```python
from build123d import *

# Parameters (mm, degrees)
SKETCH_1_W              = 150
SKETCH_1_H              = 200
EXTRUDE_1_DEPTH         = 2
CUT_EXTRUDE_1_REACH     = 127.016
SKETCH_2_R              = 2
CUT_EXTRUDE_2_REACH     = 127.016
SKETCH_3_R              = 1.6
CUT_EXTRUDE_3_REACH     = 127.016
SKETCH_5_R              = 1.6
CUT_EXTRUDE_START       = -2
CUT_EXTRUDE_4_OUTLINE_W = 150
CUT_EXTRUDE_4_OUTLINE_H = 200
CUT_EXTRUDE_4_DEPTH     = 2


# Read off the part's stored shape, not the designer's step: 切除-拉伸4
with BuildPart() as part:
    # 草图1 → 凸台-拉伸1 (new body)
    with BuildSketch(Plane(origin=(0, 0, 0), x_dir=(1, 0, 0), z_dir=(0, 1, 0))):
        Rectangle(SKETCH_1_W, SKETCH_1_H)
    extrude(amount=EXTRUDE_1_DEPTH)

    # 草图2 → 切除-拉伸1 (cut, up to next)
    with BuildSketch(Plane(origin=(0, 2, 0), x_dir=(1, 0, 0), z_dir=(0, 1, 0)), mode=Mode.PRIVATE) as cut_extrude_1_sk1:
        with Locations(Location((0, 80, 0), (0, 0, 270))):
            Circle(SKETCH_2_R)
    cut_extrude_1_tool1 = extrude(cut_extrude_1_sk1.sketch, amount=-CUT_EXTRUDE_1_REACH, mode=Mode.PRIVATE) & part.part
    add(cut_extrude_1_tool1.solids().sort_by_distance((0, 2, -80))[0], mode=Mode.SUBTRACT)

    # 草图3 → 切除-拉伸2 (cut, up to next)
    with BuildSketch(Plane(origin=(0, 2, 0), x_dir=(1, 0, 0), z_dir=(0, 1, 0)), mode=Mode.PRIVATE) as cut_extrude_2_sk1:
        with Locations(Location((-17.5, 35, 0), (0, 0, 270))):
            Circle(SKETCH_3_R)
    cut_extrude_2_tool1 = extrude(cut_extrude_2_sk1.sketch, amount=-CUT_EXTRUDE_2_REACH, mode=Mode.PRIVATE) & part.part
    # 草图3 → 切除-拉伸2 (cut, up to next)
    with BuildSketch(Plane(origin=(0, 2, 0), x_dir=(1, 0, 0), z_dir=(0, 1, 0)), mode=Mode.PRIVATE) as cut_extrude_2_sk2:
        with Locations(Location((-17.5, 25, 0), (0, 0, 90))):
            Circle(SKETCH_3_R)
    cut_extrude_2_tool2 = extrude(cut_extrude_2_sk2.sketch, amount=-CUT_EXTRUDE_2_REACH, mode=Mode.PRIVATE) & part.part
    # 草图3 → 切除-拉伸2 (cut, up to next)
    with BuildSketch(Plane(origin=(0, 2, 0), x_dir=(1, 0, 0), z_dir=(0, 1, 0)), mode=Mode.PRIVATE) as cut_extrude_2_sk3:
        with Locations(Location((17.5, 25, 0), (0, 0, 270))):
            Circle(SKETCH_3_R)
    cut_extrude_2_tool3 = extrude(cut_extrude_2_sk3.sketch, amount=-CUT_EXTRUDE_2_REACH, mode=Mode.PRIVATE) & part.part
    # 草图3 → 切除-拉伸2 (cut, up to next)
    with BuildSketch(Plane(origin=(0, 2, 0), x_dir=(1, 0, 0), z_dir=(0, 1, 0)), mode=Mode.PRIVATE) as cut_extrude_2_sk4:
        with Locations(Location((17.5, 35, 0), (0, 0, 90))):
            Circle(SKETCH_3_R)
    cut_extrude_2_tool4 = extrude(cut_extrude_2_sk4.sketch, amount=-CUT_EXTRUDE_2_REACH, mode=Mode.PRIVATE) & part.part
    add(cut_extrude_2_tool1.solids().sort_by_distance((-17.5, 2, -35))[0], mode=Mode.SUBTRACT)
    add(cut_extrude_2_tool2.solids().sort_by_distance((-17.5, 2, -25))[0], mode=Mode.SUBTRACT)
    add(cut_extrude_2_tool3.solids().sort_by_distance((17.5, 2, -25))[0], mode=Mode.SUBTRACT)
    add(cut_extrude_2_tool4.solids().sort_by_distance((17.5, 2, -35))[0], mode=Mode.SUBTRACT)

    # 草图5 → 切除-拉伸3 (cut, up to next)
    with BuildSketch(Plane(origin=(0, 2, 0), x_dir=(1, 0, 0), z_dir=(0, 1, 0)), mode=Mode.PRIVATE) as cut_extrude_3_sk1:
        with Locations(Location((32.32051615, -5, 0), (0, 0, 270))):
            Circle(SKETCH_5_R)
    cut_extrude_3_tool1 = extrude(cut_extrude_3_sk1.sketch, amount=-CUT_EXTRUDE_3_REACH, mode=Mode.PRIVATE) & part.part
    # 草图5 → 切除-拉伸3 (cut, up to next)
    with BuildSketch(Plane(origin=(0, 2, 0), x_dir=(1, 0, 0), z_dir=(0, 1, 0)), mode=Mode.PRIVATE) as cut_extrude_3_sk2:
        with Locations(Location((-32.32051615, -5, 0), (0, 0, 90))):
            Circle(SKETCH_5_R)
    cut_extrude_3_tool2 = extrude(cut_extrude_3_sk2.sketch, amount=-CUT_EXTRUDE_3_REACH, mode=Mode.PRIVATE) & part.part
    add(cut_extrude_3_tool1.solids().sort_by_distance((32.320516, 2, 5))[0], mode=Mode.SUBTRACT)
    add(cut_extrude_3_tool2.solids().sort_by_distance((-32.320516, 2, 5))[0], mode=Mode.SUBTRACT)

    # 切除-拉伸4 outline → 切除-拉伸4 (cut)
    with BuildSketch(Plane(origin=(0, 2, 0), x_dir=(1, 0, 0), z_dir=(0, 1, 0)).offset(CUT_EXTRUDE_START)):
        Rectangle(CUT_EXTRUDE_4_OUTLINE_W, CUT_EXTRUDE_4_OUTLINE_H)
        with BuildLine():
            ThreePointArc((-9.52836439, 83.034843002), (0, 90), (9.52836439, 83.034843002))
            Line((9.52836439, 83.034843002), (37.084698345, -3.482578499))
            ThreePointArc((37.084698345, -3.482578499), (36.357043587, -7.95066878), (32.32051615, -10))
            Line((32.32051615, -10), (-32.32051615, -10))
            ThreePointArc((-32.32051615, -10), (-36.357043587, -7.95066878), (-37.084698345, -3.482578499))
            Line((-37.084698345, -3.482578499), (-9.52836439, 83.034843002))
        make_face(mode=Mode.SUBTRACT)
    extrude(amount=CUT_EXTRUDE_4_DEPTH, mode=Mode.SUBTRACT)


solid = part.part
```
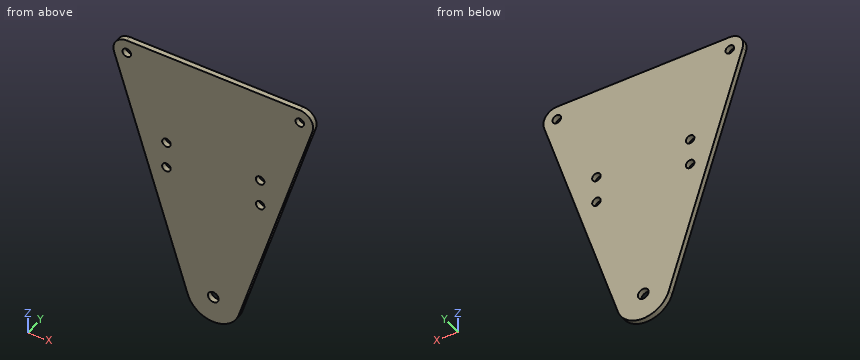
The model under review builds one solid part; all positions refer to its coordinate system, in mm. Round coordinates to 2 decimals unless told otherwise and drop trailing zeros. Write each loop counter-clockwise with the first axis right and the second up, starting at its lowest first coordinate (ties: lowest second). Pieces come first, ordered by that corner, then holes. Notation, with made-up numbers: (78.25, 51) - (88.25, 51) arc R14 ccw to (88.25, 62) - close; hole circle Ø8 at (9.5, 84). An arc over 180 degrees is marked (long way). Answer as CSV lines item,"result". Start each with the question number.
(1) We need section C-C on x = 0. State the section outline as (y, z) points, plus the area to 3 significant figures.
(2) We need section D-D on x = -17.5. State the section outline as (y, z) points.
(3) We need section A-A on y = 0.4. State the section outline as (x, z) points, plus the area to 3 significant figures.
(4) To check wall thickness, follow line 1 (X direction, y = 1.35, z = 5); line 2 (X direction, y = 0.5, z = -25); line 3 (Z direction, x = -1, y = 1.8). State the ranges of each line that lie inside material, in increasing order.
(5) We need section B-B on z = 5. State the section outline as (x, y) points, plus the area to 3 significant figures.
Worked answers:
1,outline,"(0, -90) - (2, -90) - (2, -82) - (0, -82) - close; (0, -78) - (2, -78) - (2, 10) - (0, 10) - close"
1,area,"192 mm²"
2,outline,"(0, -58.01) - (2, -58.01) - (2, -36.6) - (0, -36.6) - close; (0, -33.4) - (2, -33.4) - (2, -26.6) - (0, -26.6) - close; (0, -23.4) - (2, -23.4) - (2, 10) - (0, 10) - close"
3,outline,"(-37.08, 3.48) - (-9.53, -83.03) arc R10 ccw to (9.53, -83.03) - (37.08, 3.48) arc R5 ccw to (32.32, 10) - (-32.32, 10) arc R5 ccw to start; hole circle Ø3.2 at (-32.32, 5); hole circle Ø3.2 at (-17.5, -35); hole circle Ø3.2 at (-17.5, -25); hole circle Ø4 at (0, -80); hole circle Ø3.2 at (17.5, -35); hole circle Ø3.2 at (17.5, -25); hole circle Ø3.2 at (32.32, 5)"
3,area,"4,540 mm²"
4,line 1,"-37.32 to -33.92, -30.72 to 30.72, 33.92 to 37.32"
4,line 2,"-28.01 to -19.1, -15.9 to 15.9, 19.1 to 28.01"
4,line 3,"-89.95 to -81.73, -78.27 to 10"
5,outline,"(-37.32, 0) - (-33.92, 0) - (-33.92, 2) - (-37.32, 2) - close; (-30.72, 0) - (30.72, 0) - (30.72, 2) - (-30.72, 2) - close; (33.92, 0) - (37.32, 0) - (37.32, 2) - (33.92, 2) - close"
5,area,"136 mm²"
